from build123d import *

# Parameters (mm, degrees)
SKETCH1_W           = 101.237370502
SKETCH1_H           = 95.893480298
BOSS_EXTRUDE1_DEPTH = 5.08
CUT_EXTRUDE1_DEPTH  = 50.8
SKETCH3_W           = 34.377834067
SKETCH3_H           = 141.590062345
CUT_EXTRUDE2_DEPTH  = 25.4
SKETCH4_R           = 1.4224
CUT_EXTRUDE3_DEPTH  = 5.08


with BuildPart() as part:
    # Sketch1 → Boss-Extrude1 (new body)
    with BuildSketch(Plane.XY):
        with Locations((-50.618685251, 168.596740149)):
            Rectangle(SKETCH1_W, SKETCH1_H)
        Polygon((-101.237370502, 120.65), (0, 120.65), (0, 0), align=None)
    extrude(amount=BOSS_EXTRUDE1_DEPTH)

    # Sketch2 → Cut-Extrude1 (cut)
    with BuildSketch(Plane.XY.offset(5.08)):
        Polygon((-101.237370502, 216.543480298), (0, 108.271740149), (0, 216.543480298), align=None)
    extrude(amount=-CUT_EXTRUDE1_DEPTH, mode=Mode.SUBTRACT)

    # Sketch3 → Cut-Extrude2 (cut)
    with BuildSketch(Plane.XY.offset(5.08)):
        with Locations((5.61014441, 62.39317364)):
            Rectangle(SKETCH3_W, SKETCH3_H)
    extrude(amount=-CUT_EXTRUDE2_DEPTH, mode=Mode.SUBTRACT)

    # Sketch4 → Cut-Extrude3 (cut)
    with BuildSketch(Plane(origin=(0, 0, 0), x_dir=(0, 0, 1), z_dir=(-0.7660444431189743, -0.6427876096865437, 0))):
        with Locations(Location((2.54, 26.412934343, 0), (0, 0, 270))):
            Circle(SKETCH4_R)
        with Locations(Location((2.54, 153.412934343, 0), (0, 0, 270))):
            Circle(SKETCH4_R)
    extrude(amount=-CUT_EXTRUDE3_DEPTH, mode=Mode.SUBTRACT)


solid = part.part
Input: part model. Units: mm. Frame: model coordinates. Coordinates: 2 decimals unless noted, no trailing zeros. Order: outer loops, then holes, each group sorted by start corner. A loop starts at its lowest first (then second) coordinate and runs counter-clockwise, first axis right, second up.
1. Ray query, line 1 along Y through (x, z) = (-97.5, 3.5); line 2 along X through (y, z) = (95.5, 0.3); line 3 along Y through (x, z) = (-41, 3.4). Return the intervals inside material, ascending.
Checked values:
line 1: y = 116.2 to 117.08, 119.82 to 212.55
line 2: x = -80.13 to -11.58
line 3: y = 48.86 to 152.12
2. Cut plane B-B, the plane x = -27. Return loops of the section in (y, z).
Checked values:
outline: (32.18, 0) - (137.15, 0) - (137.15, 5.08) - (32.18, 5.08) - close
3. Draft query along X for faces 1 (the flat face through (-57, 117, 5.08)), 2 (the flat face through (-11.579, 66, 3)), 3 (the cylindrical face through (-95.85, 118.12, 2)). Return one class per face: +X half, -X half, draft (parallel to the pull), parting line (faces both ways), or undercut.
Checked values:
face 1: draft
face 2: +X half
face 3: undercut
4. Cut plane A-A, the plane y = 186. Return loops of the section in (x, z), plus the area to 3 significant figures.
Checked values:
outline: (-101.24, 0) - (-72.68, 0) - (-72.68, 5.08) - (-101.24, 5.08) - close
area: 145 mm2
